Here's how the part is built. I have some questions about the finished solid (model axes, mm). A direction names the side the tool comes from. Round coordinates to 2 decimals unless told otherwise and drop trailing zeros. Order: outer loops, then holes, each group sorted by start corner. A loop starts at its lowest first (then second) coordinate and runs counter-clockwise, first axis right, second up. Notation, with made-up numbers: M -14.5,-25.75 L 14.5,-25.75 A17 ccw 14.5,-15.75 Z; hole C 48,61 d7. An arc over 180 degrees is marked long. Write item = value, one per line. Start each with the question number.
Item 1: I want a section at C-C, the plane x = -60.5. List the corners of the cut face in (y, z) for me, plus the area to 3 significant figures.
Item 2: I want a section at D-D, the plane z = -19.5. List the corners of the cut face in (x, y) for me.
Item 3: I'm going to push flat-ended pins straight in: P1, Ø3, axis at y = 12.5, z = -19.5, coming from the +X side; P2, Ø1.5, axis at y = 15, z = -13, coming from the -X side. Where does each tip first touch, or does it pass through?
Item 4: For faces 1 (the face through (-21, 10, -16.2)), 2 (the face through (-39, 0, 2)), 3 (the face through (-55, 10, -18.6)), which set-ups out of +Z, -Z, +X, -X, +Y, -Y let a thin tool reach every point of the face, with its end or its side?
Item 5: Please list where these lines run through material, in increasing order: L1, parallel to Z at x = -61, y = 3.25; L2, parallel to Z at x = -17.5, y = 3.5; L3, parallel to X at y = 14, z = -17.
Item 6: I want a section at A-A, the plane x = -20. List the corners of the cut face in (y, z) for me, plus the area to 3 significant figures.
Item 7: I want a section at B-B, the plane y = 8.75. List the corners of the cut face in (x, z) for me.
Autodesk Inventor part; units mm, degrees
ref_plane "YZ Plane" through (0, 0, 0) normal (1, 0, 0) x (0, 1, 0)
ref_plane "XZ Plane" through (0, 0, 0) normal (0, 1, 0) x (-1, 0, 0)
ref_plane "XY Plane" through (0, 0, 0) normal (0, 0, 1) x (1, 0, 0)
sketch "Skizze1" plane through (0, 0, 0) normal (0, 1, 0) x (-1, 0, 0)
  arc A0 (4, -6.9282) -> (0, 8) centre (0, 0) ccw
  line L0 (0, -22) -> (0, -27)
  line L1 (0, -27) -> (30, -27)
  line L2 (80, 8) -> (0, 8)
  line L3 (0, -22) -> (25, -22)
  line L4 (25, -22) -> (0, -22)
  line L5 (25, -22) -> (25, -16.2)
  line L6 (25, -16) -> (25, -22)
  line L7 (25, -16.2) -> (16.7663, -16.2)
  line L8 (16.7663, -16.2) -> (4, -6.9282)
  line L9 (30, -27) -> (80, -27)
  line L10 (80, -27) -> (80, -18.6)
  line L11 (80, -18.6) -> (30, -18.6)
  line L12 (80, 8) -> (80, 1.45)
  line L13 (80, 1.45) -> (30, 1.45)
  line L14 (30, -18.6) -> (30, 1.45)
  dimension "d0" = 5
  dimension "d9" = 50
  dimension "d10" = 8.4
  dimension "d12" = 20.05
extrude "Extrusion1" add sketch "Skizze1" along normal blind 20
properties part number "Halterung_MobileWhiteboard_V3"
Filled in:
q1.outline = M 0,-27 L 20,-27 L 20,-18.6 L 0,-18.6 Z; M 0,1.45 L 20,1.45 L 20,8 L 0,8 Z
q1.area = 299 mm^2
q2.outline = M -80,0 L -25,0 L -25,20 L -80,20 Z
q3.P1 = -25
q3.P2 = -30
q4.face_1 = +X, +Y, -Y
q4.face_2 = +Z, -Z, +X, -X, -Y
q4.face_3 = -X, +Y, -Y
q5.L1 = -27 to -18.6, 1.45 to 8
q5.L2 = -27 to -22, -16.2 to 8
q5.L3 = -30 to -25
q6.outline = M 0,-27 L 20,-27 L 20,-22 L 0,-22 Z; M 0,-16.2 L 20,-16.2 L 20,8 L 0,8 Z
q6.area = 584 mm^2
q7.outline = M -80,-27 L 0,-27 L 0,-22 L -25,-22 L -25,-16.2 L -16.77,-16.2 L -4,-6.93 A8 cw 0,8 L -80,8 L -80,1.45 L -30,1.45 L -30,-18.6 L -80,-18.6 Z
